```python
from build123d import *

# Parameters (mm, degrees)
SKETCH1_R           = 1.5
SKETCH1_R_2         = 12.095
SKETCH1_R_3         = 1.143
BOSS_EXTRUDE2_DEPTH = 3.175


with BuildPart() as part:
    # Sketch1 → Boss-Extrude2 (new body)
    with BuildSketch(Plane(origin=(0, 0, 0), x_dir=(1, 0, 0), z_dir=(0, 1, 0))):
        with BuildLine():
            ThreePointArc((31.589980006, -65.102164912), (33.357679643, -66.33740492), (35.49727084, -66.067721036))
            ThreePointArc((35.49727084, -66.067721036), (0, 75), (-35.49727084, -66.067721036))
            ThreePointArc((-35.49727084, -66.067721036), (-33.357679643, -66.33740492), (-31.589980006, -65.102164912))
            ThreePointArc((-31.589980006, -65.102164912), (0, -48.302004425), (31.589980006, -65.102164912))
        make_face()
        with Locations((-33.059737365, -55.383244446)):
            Circle(SKETCH1_R, mode=Mode.SUBTRACT)
        with Locations((-23.852486199, -41.694616163)):
            Circle(SKETCH1_R, mode=Mode.SUBTRACT)
        with Locations((0, -39.659190322)):
            Circle(SKETCH1_R, mode=Mode.SUBTRACT)
        with Locations((-40.277379234, -25.14022965)):
            Circle(SKETCH1_R, mode=Mode.SUBTRACT)
        with BuildLine():
            Line((-52.910067426, -34.5), (-64.910067426, -34.5))
            ThreePointArc((-64.910067426, -34.5), (-65.263620817, -34.353553391), (-65.410067426, -34))
            Line((-65.410067426, -34), (-65.410067426, 34))
            ThreePointArc((-65.410067426, 34), (-65.263620817, 34.353553391), (-64.910067426, 34.5))
            Line((-64.910067426, 34.5), (-52.910067426, 34.5))
            ThreePointArc((-52.910067426, 34.5), (-52.556514035, 34.353553391), (-52.410067426, 34))
            Line((-52.410067426, 34), (-52.410067426, -34))
            ThreePointArc((-52.410067426, -34), (-52.556514035, -34.353553391), (-52.910067426, -34.5))
        make_face(mode=Mode.SUBTRACT)
        with Locations((-41.910067426, -11.1)):
            Circle(SKETCH1_R, mode=Mode.SUBTRACT)
        with Locations((-27.645294552, -18.614761308)):
            Circle(SKETCH1_R_2, mode=Mode.SUBTRACT)
        with Locations((0, -25.409190322)):
            Circle(SKETCH1_R_2, mode=Mode.SUBTRACT)
        with Locations((-13.608916499, -21.183093811)):
            Circle(SKETCH1_R, mode=Mode.SUBTRACT)
        with Locations((-10.160067426, -11.1)):
            Circle(SKETCH1_R, mode=Mode.SUBTRACT)
        with Locations((33.059737365, -55.383244446)):
            Circle(SKETCH1_R, mode=Mode.SUBTRACT)
        with Locations((23.852486199, -41.694616163)):
            Circle(SKETCH1_R, mode=Mode.SUBTRACT)
        with Locations((13.608916499, -21.183093811)):
            Circle(SKETCH1_R, mode=Mode.SUBTRACT)
        with Locations((27.645294552, -18.614761308)):
            Circle(SKETCH1_R_2, mode=Mode.SUBTRACT)
        with Locations((10.160067426, -11.1)):
            Circle(SKETCH1_R, mode=Mode.SUBTRACT)
        with Locations((40.277379234, -25.14022965)):
            Circle(SKETCH1_R, mode=Mode.SUBTRACT)
        with Locations((41.910067426, -11.1)):
            Circle(SKETCH1_R, mode=Mode.SUBTRACT)
        with BuildLine():
            ThreePointArc((52.910067426, -34.5), (52.556514035, -34.353553391), (52.410067426, -34))
            Line((52.410067426, -34), (52.410067426, 34))
            ThreePointArc((52.410067426, 34), (52.556514035, 34.353553391), (52.910067426, 34.5))
            Line((52.910067426, 34.5), (64.910067426, 34.5))
            ThreePointArc((64.910067426, 34.5), (65.263620817, 34.353553391), (65.410067426, 34))
            Line((65.410067426, 34), (65.410067426, -34))
            ThreePointArc((65.410067426, -34), (65.263620817, -34.353553391), (64.910067426, -34.5))
            Line((64.910067426, -34.5), (52.910067426, -34.5))
        make_face(mode=Mode.SUBTRACT)
        with Locations((-41.910067426, 11.1)):
            Circle(SKETCH1_R, mode=Mode.SUBTRACT)
        with Locations((-46.011477091, 28.075890486)):
            Circle(SKETCH1_R, mode=Mode.SUBTRACT)
        with Locations((-19.397913834, 18.186588214)):
            Circle(SKETCH1_R, mode=Mode.SUBTRACT)
        with Locations((-10.160067426, 11.1)):
            Circle(SKETCH1_R, mode=Mode.SUBTRACT)
        with Locations((0, 15.543589551)):
            Circle(SKETCH1_R, mode=Mode.SUBTRACT)
        with Locations((-32.272094543, 24.295431891)):
            Circle(SKETCH1_R_2, mode=Mode.SUBTRACT)
        with Locations((-26.163250867, 37.1696126)):
            Circle(SKETCH1_R, mode=Mode.SUBTRACT)
        with Locations((0, 29.793589551)):
            Circle(SKETCH1_R_2, mode=Mode.SUBTRACT)
        with Locations((-33.059737365, 55.383244446)):
            Circle(SKETCH1_R, mode=Mode.SUBTRACT)
        with Locations((-20.05440719, 50.04379331)):
            Circle(SKETCH1_R_2, mode=Mode.SUBTRACT)
        with Locations((-10.027203595, 39.91869143)):
            Circle(SKETCH1_R, mode=Mode.SUBTRACT)
        with Locations((-6.731, 61.422565207)):
            Circle(SKETCH1_R_3, mode=Mode.SUBTRACT)
        with Locations((10.160067426, 11.1)):
            Circle(SKETCH1_R, mode=Mode.SUBTRACT)
        with Locations((19.397913834, 18.186588214)):
            Circle(SKETCH1_R, mode=Mode.SUBTRACT)
        with Locations((32.272094543, 24.295431891)):
            Circle(SKETCH1_R_2, mode=Mode.SUBTRACT)
        with Locations((26.163250867, 37.1696126)):
            Circle(SKETCH1_R, mode=Mode.SUBTRACT)
        with Locations((41.910067426, 11.1)):
            Circle(SKETCH1_R, mode=Mode.SUBTRACT)
        with Locations((46.011477091, 28.075890486)):
            Circle(SKETCH1_R, mode=Mode.SUBTRACT)
        with Locations((10.027203595, 39.91869143)):
            Circle(SKETCH1_R, mode=Mode.SUBTRACT)
        with Locations((20.05440719, 50.04379331)):
            Circle(SKETCH1_R_2, mode=Mode.SUBTRACT)
        with Locations((33.059737365, 55.383244446)):
            Circle(SKETCH1_R, mode=Mode.SUBTRACT)
        with Locations((6.731, 61.422565207)):
            Circle(SKETCH1_R_3, mode=Mode.SUBTRACT)
    extrude(amount=BOSS_EXTRUDE2_DEPTH)


solid = part.part
```
Design review of the part built by this model. Coordinates are the model's own, in mm. A direction names the side the tool comes from. Give positions to 0.01 mm unless a question says otherwise; leave off trailing zeros. Order: outer loops, then holes, each group sorted by start corner. A loop starts at its lowest first (then second) coordinate and runs counter-clockwise, first axis right, second up. Notation, with made-up numbers: M -11.5,79.25 L 16.5,79.25 A22 ccw 16.5,96.25 Z; hole C 76,-37.75 d5. An arc over 180 degrees is marked long. One line per question, with ' | ' between items. Start each with the question number.
Q1. We need section B-B (y = 2.45). State how many separate pieces and enclosed holes the cut face has, plus the area to 3 significant figures.
Q2. Machinability: for faces 1 (the face through (-33.388, 1.565, 66.345)), 2 (the face through (59, 2, 34.5)), which of the approach directions +Z, -Z, +X, -X, +Y, -Y give a long, thin tool a straight path to every point of the face, cutting with its end or side? Answer none if there is none.
Q3. The part is to be moulded in two halves that separate along X. For faces 3 (the face through (22.7, 1.6, -16.9)), 4 (the face through (-1, 3.175, -5)), 5 (the face through (2.78, 1.57, -74.95)), say which applies: +X half, -X half, draft (parallel to the pull), parting line (faces both ways), or undercut.
Q4. For pin 1 Ø1 at (x, y) = (-60.5, 1) entering from -Z; pin 2 Ø1 at (y, z) = (2, 35.5) entering from -X; pin 3 Ø1.6 at (x, y) = (57, 1.5) entering from +Z, all flat-tipped, find the tip position at first contact; note any pin that passes through.
Q5. For L1, parallel to X at y = 1.95, z = -48.5; L2, parallel to X at y = 0.85, z = -39.5; L3, parallel to Z at x = -27.5, y = 0.3, list the stretches that pass through material, from the lowest coordinate up. Write a range as [from, to].
Q6. We need section A-A (z = 0). Write out the cut boundary in (x, y) (3 decimals), plus the area to 3 significant figures.
Returned:
1) separate pieces: 1 | enclosed holes: 40 | area: 10,800 mm2
2) face 1: +Z, +Y, -Y | face 2: +Y, -Y
3) face 3: undercut | face 4: draft | face 5: parting line
4) pin 1: z = -45 | pin 2: x = -66.33 | pin 3: z = 49.66
5) L1: [-57.21, -32.05], [-8.06, 8.06], [32.05, 57.21] | L2: [-63.76, -25.98], [-14.13, -11.47], [-8.59, -7.22], [7.22, 8.59], [11.47, 14.13], [25.98, 63.76] | L3: [-69.78, -59.58], [-40.51, -37.85], [-36.49, -35.41], [-13.18, 6.52], [30.71, 60.03]
6) outline: M -75,0 L -65.41,0 L -65.41,3.175 L -75,3.175 Z; M -52.41,0 L 52.41,0 L 52.41,3.175 L -52.41,3.175 Z; M 65.41,0 L 75,0 L 75,3.175 L 65.41,3.175 Z | area: 394 mm2
